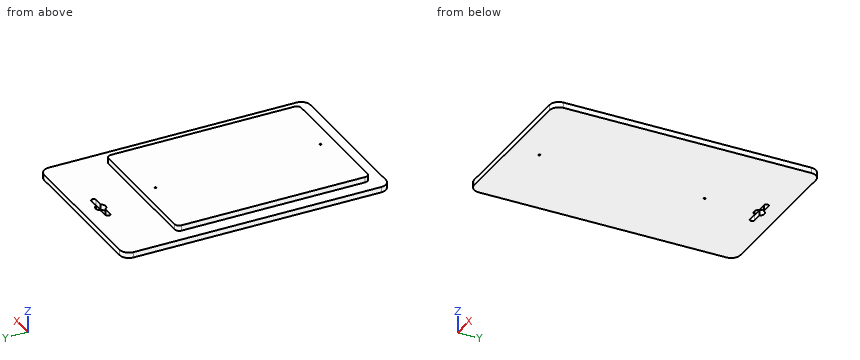
from build123d import *

# Parameters (mm, degrees)
F1_DEPTH  = 6
F2_W      = 180
F2_H      = 240
F3_DEPTH  = 6
F4_W      = 180
F4_H      = 50
F5_DEPTH  = 6
F6_R      = 10.1
F8_DEPTH  = 25
F9_R      = 1
F10_DEPTH = 25


with BuildPart() as f1:
    # F0 (on Top) → F1 (new body)
    with BuildSketch(Plane.XY):
        with BuildLine():
            ThreePointArc((75, 100), (73.5355339059, 103.5355339059), (70, 105))
            Line((70, 105), (-70, 105))
            ThreePointArc((-70, 105), (-73.5355339059, 103.5355339059), (-75, 100))
            Line((-75, 100), (-75, -100))
            ThreePointArc((-75, -100), (-73.5355339059, -103.5355339059), (-70, -105))
            Line((-70, -105), (70, -105))
            ThreePointArc((70, -105), (73.5355339059, -103.5355339059), (75, -100))
            Line((75, -100), (75, 100))
        make_face()
    extrude(amount=F1_DEPTH)

    # F2 (on face) → F3 (join)
    with BuildSketch(Plane(origin=(0, 0, 0), x_dir=(1, 0, 0), z_dir=(0, 0, -1))):
        Rectangle(F2_W, F2_H)
        with BuildLine():
            ThreePointArc((75, -100), (73.5355339059, -103.5355339059), (70, -105))
            Line((70, -105), (-70, -105))
            ThreePointArc((-70, -105), (-73.5355339059, -103.5355339059), (-75, -100))
            Line((-75, -100), (-75, 100))
            ThreePointArc((-75, 100), (-73.5355339059, 103.5355339059), (-70, 105))
            Line((-70, 105), (70, 105))
            ThreePointArc((70, 105), (73.5355339059, 103.5355339059), (75, 100))
            Line((75, 100), (75, -100))
        make_face(mode=Mode.SUBTRACT)
        with BuildLine():
            Line((-70, -105), (70, -105))
            ThreePointArc((70, -105), (73.5355339059, -103.5355339059), (75, -100))
            Line((75, -100), (75, 100))
            ThreePointArc((75, 100), (73.5355339059, 103.5355339059), (70, 105))
            Line((70, 105), (-70, 105))
            ThreePointArc((-70, 105), (-73.5355339059, 103.5355339059), (-75, 100))
            Line((-75, 100), (-75, -100))
            ThreePointArc((-75, -100), (-73.5355339059, -103.5355339059), (-70, -105))
        make_face()
    extrude(amount=F3_DEPTH)

    # F4 (on face) → F5 (join)
    with BuildSketch(Plane.XY):
        with Locations((0, 145)):
            Rectangle(F4_W, F4_H)
    extrude(amount=-F5_DEPTH)

    # F6
    f6_edges = [f1.edges().sort_by_distance(p)[0] for p in [
        (-90, 170, -3),
        (90, 170, -3),
        (-90, -120, -3),
        (90, -120, -3),
    ]]
    fillet(f6_edges, radius=F6_R)

    # F7 (on face) → F8 (cut)
    with BuildSketch(Plane.XY):
        with BuildLine():
            ThreePointArc((4.8989794856, 147), (5.3476343915, 148.2143848108), (5.5, 149.5))
            ThreePointArc((5.5, 149.5), (5.3476343915, 150.7856151892), (4.8989794856, 152))
            Line((4.8989794856, 152), (-4.8989794856, 152))
            ThreePointArc((-4.8989794856, 152), (-5.5, 149.5), (-4.8989794856, 147))
            Line((-4.8989794856, 147), (4.8989794856, 147))
        make_face()
        with BuildLine():
            ThreePointArc((4.8989794856, 152), (5.3476343915, 150.7856151892), (5.5, 149.5))
            ThreePointArc((5.5, 149.5), (5.3476343915, 148.2143848108), (4.8989794856, 147))
            Line((4.8989794856, 147), (15, 147))
            ThreePointArc((15, 147), (16.767766953, 147.732233047), (17.5, 149.5))
            ThreePointArc((17.5, 149.5), (16.767766953, 151.267766953), (15, 152))
            Line((15, 152), (4.8989794856, 152))
        make_face()
        with BuildLine():
            Line((-4.8989794856, 152), (4.8989794856, 152))
            ThreePointArc((4.8989794856, 152), (0, 155), (-4.8989794856, 152))
        make_face()
        with BuildLine():
            ThreePointArc((-4.8989794856, 147), (0, 144), (4.8989794856, 147))
            Line((4.8989794856, 147), (-4.8989794856, 147))
        make_face()
        with BuildLine():
            ThreePointArc((-4.8989794856, 147), (-5.5, 149.5), (-4.8989794856, 152))
            Line((-4.8989794856, 152), (-15, 152))
            ThreePointArc((-15, 152), (-16.767766953, 151.267766953), (-17.5, 149.5))
            ThreePointArc((-17.5, 149.5), (-16.767766953, 147.732233047), (-15, 147))
            Line((-15, 147), (-4.8989794856, 147))
        make_face()
    extrude(amount=-F8_DEPTH, mode=Mode.SUBTRACT)

    # F9 (on face) → F10 (cut)
    with BuildSketch(Plane.XY.offset(6)):
        with Locations((0, 90)):
            Circle(F9_R)
        with Locations((0, -90)):
            Circle(F9_R)
    extrude(amount=-F10_DEPTH, mode=Mode.SUBTRACT)


solid = f1.part
Read the model definition and answer for the solid it produces. Units are mm, in the model's axes. Give positions to 0.01 mm unless a question says otherwise; leave off trailing zeros. Loops run counter-clockwise (first coordinate to the right, second up) from the corner with the lowest first, then second, coordinate; pieces in that order, holes last. Notation, with made-up numbers: (-10, 26) -> (9, 26) arc R24 ccw to (9, 44) -> close; hole circle Ø11 at (-19.75, 62.25). An arc over 180 degrees is marked (long way). Answer as CSV lines item,"result".
Item 1: Each of these flat-tipped pins is pushed along its axis until it touches: pin 1 (2 mm diameter, centred on x = -68.5, y = 114, fed in from +Z); pin 2 (1.8 mm diameter, centred on x = 0, y = -90, fed in from -Z). Where does it stop, or does it pass through?
Returned:
pin 1,"stops at z = 0"
pin 2,"passes through"
Item 2: Consider line 1 (Y direction, x = 0, z = 2.25); line 2 (X direction, y = -90, z = 2.5); line 3 (X direction, y = -90, z = -3.5). Determine where each line is inside the solid, lowest interval first. Write a range as [from, to].
Returned:
line 1,"y = [-105, -91], [-89, 89], [91, 105]"
line 2,"x = [-75, -1], [1, 75]"
line 3,"x = [-90, -1], [1, 90]"
Item 3: Find section C-C on y = -34.5. Give the vertices of the cut face in (x, z), plus the area to 3 significant figures.
Returned:
outline,"(-90, -6) -> (90, -6) -> (90, 0) -> (75, 0) -> (75, 6) -> (-75, 6) -> (-75, 0) -> (-90, 0) -> close"
area,"1,980 mm²"
Item 4: Find section A-A on x = -9. Give the vertices of the cut face in (y, z), plus the area to 3 significant figures.
Returned:
outline,"(-120, -6) -> (147, -6) -> (147, 0) -> (105, 0) -> (105, 6) -> (-105, 6) -> (-105, 0) -> (-120, 0) -> close; (152, -6) -> (170, -6) -> (170, 0) -> (152, 0) -> close"
area,"2,970 mm²"
Item 5: Find section B-B on x = -34. Give the vertices of the cut face in (y, z).
Returned:
outline,"(-120, -6) -> (170, -6) -> (170, 0) -> (105, 0) -> (105, 6) -> (-105, 6) -> (-105, 0) -> (-120, 0) -> close"
